Part print with two shaded views. Sizes in mm from the minimum x, y, z corner. A direction names the side the tool comes from. Coordinates: 2 decimals unless noted, no trailing zeros. Loops run counter-clockwise (first coordinate to the right, second up) from the corner with the lowest first, then second, coordinate; pieces in that order, holes last.
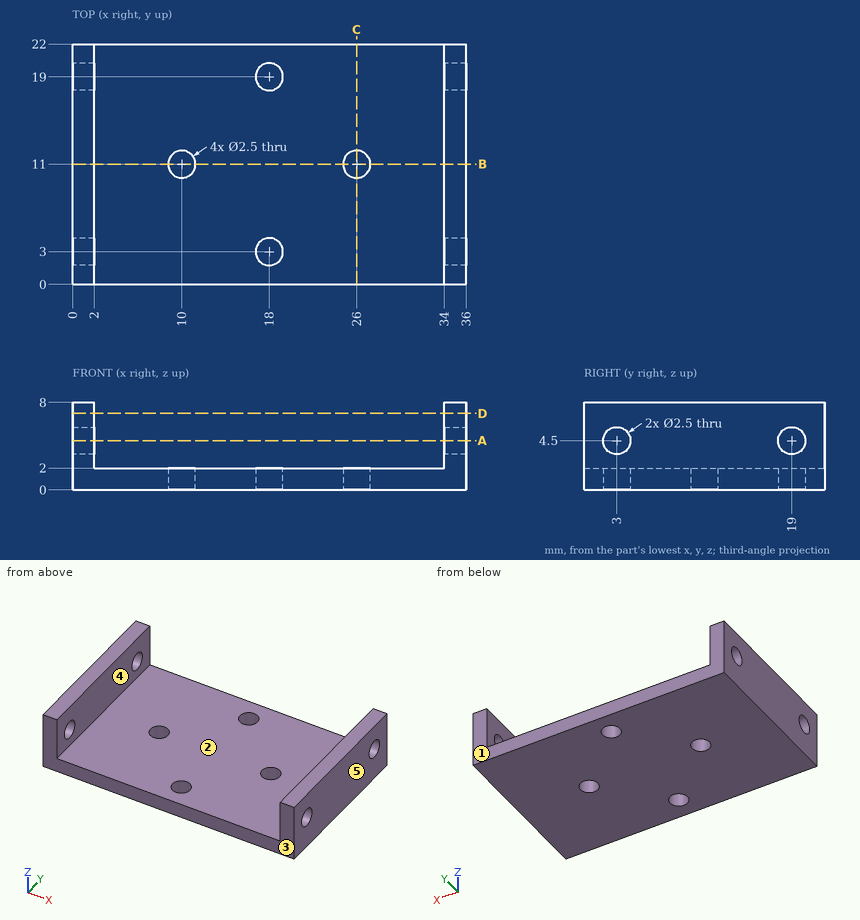
Q1. Slice it at B-B (y = 11). List the corners of the cut face in (x, z), and give its area (3 significant figures).
Answers:
outline: (0, 0) - (8.75, 0) - (8.75, 2) - (2, 2) - (2, 8) - (0, 8) - close; (11.25, 0) - (24.75, 0) - (24.75, 2) - (11.25, 2) - close; (27.25, 0) - (36, 0) - (36, 8) - (34, 8) - (34, 2) - (27.25, 2) - close
area: 86.0 mm2
Q2. Slice it at A-A (z = 4.5). List the corners of the cut face in (x, y).
Answers:
outline: (0, 0) - (2, 0) - (2, 1.75) - (0, 1.75) - close; (0, 4.25) - (2, 4.25) - (2, 17.75) - (0, 17.75) - close; (0, 20.25) - (2, 20.25) - (2, 22) - (0, 22) - close; (34, 0) - (36, 0) - (36, 1.75) - (34, 1.75) - close; (34, 4.25) - (36, 4.25) - (36, 17.75) - (34, 17.75) - close; (34, 20.25) - (36, 20.25) - (36, 22) - (34, 22) - close
Q3. Flat gauge pin, fed straight in: P1, Ø5, axis at x = 9.5, y = 5, coming from the +Z side. Where does the tip first touch, or does it go through?
Answers:
P1: stops at z = 2
Q4. Slice it at D-D (z = 7). List the corners of the cut face in (x, y).
Answers:
outline: (0, 0) - (2, 0) - (2, 22) - (0, 22) - close; (34, 0) - (36, 0) - (36, 22) - (34, 22) - close
Q5. Which spindle directions (+Z, -Z, +X, -X, +Y, -Y) get a long thin tool onto all of the face, cutting with end or side? Do the marked faces 1 and 2. Say none if no direction does.
Answers:
face 1: +Z, -Z, +X, -X, +Y
face 2: +Z, +Y, -Y
Q6. Drill centre lines: line 1 (Y direction, x = 18, z = 0.75); line 2 (X direction, y = 10.25, z = 1.75); line 3 (X direction, y = 15.5, z = 6.25). Where is each one in solid material? Low to high.
Answers:
line 1: y = 0 to 1.75, 4.25 to 17.75, 20.25 to 22
line 2: x = 0 to 9, 11 to 25, 27 to 36
line 3: x = 0 to 2, 34 to 36
Q7. Slice it at C-C (x = 26). List the corners of the cut face in (y, z), and give its area (3 significant figures).
Answers:
outline: (0, 0) - (9.75, 0) - (9.75, 2) - (0, 2) - close; (12.25, 0) - (22, 0) - (22, 2) - (12.25, 2) - close
area: 39.0 mm2
Q8. Mould opens along X. For the marked faces 3, 4 and 5 say: +X half, -X half, draft (parallel to the pull), parting line (faces both ways), or undercut.
Answers:
face 3: draft
face 4: undercut
face 5: +X half
